Read the model definition and answer for the solid it produces. Units are mm, in the model's axes. A direction names the side the tool comes from. Round coordinates to 2 decimals unless told otherwise and drop trailing zeros. Loops run counter-clockwise (first coordinate to the right, second up) from the corner with the lowest first, then second, coordinate; pieces in that order, holes last. Notation, with made-up numbers: M 85.5,12.5 L 94.5,12.5 A18 cw 94.5,25.5 Z; hole C 38,68.5 d9. An arc over 180 degrees is marked long. Write each question's results on one line, items separated by ' | '.
from build123d import *

# Parameters (mm, degrees)
SKETCH1_R                = 14.5
BOSS_EXTRUDE1_DEPTH      = 4
BOSS_EXTRUDE2_DEPTH      = 2
BOSS_EXTRUDE2_DEPTH_BACK = 125
SKETCH2_R                = 5
SKETCH2_R_2              = 4
SKETCH2_R_3              = 3.453892414
SKETCH2_R_4              = 2.453892414
LPATTERN4_START          = -124
LPATTERN4_OUTLINE_R      = 14.5
LPATTERN4_DEPTH          = 4
LPATTERN4_START_2        = -62
LPATTERN4_2_OUTLINE_R    = 14.5
LPATTERN4_2_OUTLINE_R_2  = 3.453892414
LPATTERN4_2_OUTLINE_R_3  = 5
LPATTERN4_2_OUTLINE_R_4  = 4
LPATTERN4_2_OUTLINE_R_5  = 2.453892414
LPATTERN4_2_DEPTH        = 4
SKETCH8_R                = 2.453892414
CUT_EXTRUDE4_DEPTH       = 128
SKETCH12_R               = 2.875
BOSS_EXTRUDE4_DEPTH      = 41
CUT_EXTRUDE5_DEPTH       = 41
SKETCH14_R               = 4
CUT_EXTRUDE6_DEPTH       = 124


# Read off the part's stored shape, not the designer's step: LPattern4
with BuildPart() as part:
    # Sketch1 → Boss-Extrude1 (new body)
    with BuildSketch(Plane(origin=(0, 0, 0), x_dir=(1, 0, 0), z_dir=(0, 1, 0))):
        with Locations(Location((0, 0, 0), (0, 0, 270))):
            Circle(SKETCH1_R)
    extrude(amount=BOSS_EXTRUDE1_DEPTH)

    # Sketch2 → Boss-Extrude2 (add, two sides: drawn at the far end of the back side and taken through both)
    # profile 1 of 7: a face of its own
    with BuildSketch(Plane(origin=(0, 4, 0), x_dir=(1, 0, 0), z_dir=(0, 1, 0)).offset(-BOSS_EXTRUDE2_DEPTH_BACK)):
        with Locations(Location((0, 0, 0), (0, 0, 270))):
            Circle(SKETCH2_R)
        with Locations(Location((0, 0, 0), (0, 0, 270))):
            Circle(SKETCH2_R_2, mode=Mode.SUBTRACT)
    # profile 2 of 7: a face of its own
    with BuildSketch(Plane(origin=(0, 4, 0), x_dir=(1, 0, 0), z_dir=(0, 1, 0)).offset(-BOSS_EXTRUDE2_DEPTH_BACK)):
        with Locations(Location((0, 9.4, 0), (0, 0, 270))):
            Circle(SKETCH2_R_3)
        with Locations(Location((0, 9.4, 0), (0, 0, 270))):
            Circle(SKETCH2_R_4, mode=Mode.SUBTRACT)
    # profile 3 of 7: a face of its own
    with BuildSketch(Plane(origin=(0, 4, 0), x_dir=(1, 0, 0), z_dir=(0, 1, 0)).offset(-BOSS_EXTRUDE2_DEPTH_BACK)):
        with Locations(Location((8.140638796, 4.7, 0), (0, 0, 270))):
            Circle(SKETCH2_R_3)
        with Locations(Location((8.140638796, 4.7, 0), (0, 0, 270))):
            Circle(SKETCH2_R_4, mode=Mode.SUBTRACT)
    # profile 4 of 7: a face of its own
    with BuildSketch(Plane(origin=(0, 4, 0), x_dir=(1, 0, 0), z_dir=(0, 1, 0)).offset(-BOSS_EXTRUDE2_DEPTH_BACK)):
        with Locations(Location((8.140638796, -4.7, 0), (0, 0, 270))):
            Circle(SKETCH2_R_3)
        with Locations(Location((8.140638796, -4.7, 0), (0, 0, 270))):
            Circle(SKETCH2_R_4, mode=Mode.SUBTRACT)
    # profile 5 of 7: a face of its own
    with BuildSketch(Plane(origin=(0, 4, 0), x_dir=(1, 0, 0), z_dir=(0, 1, 0)).offset(-BOSS_EXTRUDE2_DEPTH_BACK)):
        with Locations(Location((0, -9.4, 0), (0, 0, 270))):
            Circle(SKETCH2_R_3)
        with Locations(Location((0, -9.4, 0), (0, 0, 270))):
            Circle(SKETCH2_R_4, mode=Mode.SUBTRACT)
    # profile 6 of 7: a face of its own
    with BuildSketch(Plane(origin=(0, 4, 0), x_dir=(1, 0, 0), z_dir=(0, 1, 0)).offset(-BOSS_EXTRUDE2_DEPTH_BACK)):
        with Locations(Location((-8.140638796, -4.7, 0), (0, 0, 270))):
            Circle(SKETCH2_R_3)
        with Locations(Location((-8.140638796, -4.7, 0), (0, 0, 270))):
            Circle(SKETCH2_R_4, mode=Mode.SUBTRACT)
    # profile 7 of 7: a face of its own
    with BuildSketch(Plane(origin=(0, 4, 0), x_dir=(1, 0, 0), z_dir=(0, 1, 0)).offset(-BOSS_EXTRUDE2_DEPTH_BACK)):
        with Locations(Location((-8.140638796, 4.7, 0), (0, 0, 270))):
            Circle(SKETCH2_R_3)
        with Locations(Location((-8.140638796, 4.7, 0), (0, 0, 270))):
            Circle(SKETCH2_R_4, mode=Mode.SUBTRACT)
    extrude(amount=BOSS_EXTRUDE2_DEPTH + BOSS_EXTRUDE2_DEPTH_BACK)

    # LPattern4 outline → LPattern4 (add)
    with BuildSketch(Plane(origin=(0, 0, 0), x_dir=(1, 0, 0), z_dir=(0, 1, 0)).offset(LPATTERN4_START)):
        Circle(LPATTERN4_OUTLINE_R)
    extrude(amount=LPATTERN4_DEPTH)

    # LPattern4 2 outline → LPattern4 2 (add)
    # profile 1 of 8: a face of its own
    with BuildSketch(Plane(origin=(0, 0, 0), x_dir=(1, 0, 0), z_dir=(0, 1, 0)).offset(LPATTERN4_START_2)):
        Circle(LPATTERN4_2_OUTLINE_R)
        with Locations((-8.140638796, -4.7)):
            Circle(LPATTERN4_2_OUTLINE_R_2, mode=Mode.SUBTRACT)
        with Locations((0, -9.4)):
            Circle(LPATTERN4_2_OUTLINE_R_2, mode=Mode.SUBTRACT)
        with Locations((8.140638796, -4.7)):
            Circle(LPATTERN4_2_OUTLINE_R_2, mode=Mode.SUBTRACT)
        with Locations((-8.140638796, 4.7)):
            Circle(LPATTERN4_2_OUTLINE_R_2, mode=Mode.SUBTRACT)
        Circle(LPATTERN4_2_OUTLINE_R_3, mode=Mode.SUBTRACT)
        with Locations((8.140638796, 4.7)):
            Circle(LPATTERN4_2_OUTLINE_R_2, mode=Mode.SUBTRACT)
        with Locations((0, 9.4)):
            Circle(LPATTERN4_2_OUTLINE_R_2, mode=Mode.SUBTRACT)
    # profile 2 of 8: a face of its own
    with BuildSketch(Plane(origin=(0, 0, 0), x_dir=(1, 0, 0), z_dir=(0, 1, 0)).offset(LPATTERN4_START_2)):
        Circle(LPATTERN4_2_OUTLINE_R_4)
    # profile 3 of 8: a face of its own
    with BuildSketch(Plane(origin=(0, 0, 0), x_dir=(1, 0, 0), z_dir=(0, 1, 0)).offset(LPATTERN4_START_2)):
        with Locations((0, 9.4)):
            Circle(LPATTERN4_2_OUTLINE_R_5)
    # profile 4 of 8: a face of its own
    with BuildSketch(Plane(origin=(0, 0, 0), x_dir=(1, 0, 0), z_dir=(0, 1, 0)).offset(LPATTERN4_START_2)):
        with Locations((8.140638796, 4.7)):
            Circle(LPATTERN4_2_OUTLINE_R_5)
    # profile 5 of 8: a face of its own
    with BuildSketch(Plane(origin=(0, 0, 0), x_dir=(1, 0, 0), z_dir=(0, 1, 0)).offset(LPATTERN4_START_2)):
        with Locations((8.140638796, -4.7)):
            Circle(LPATTERN4_2_OUTLINE_R_5)
    # profile 6 of 8: a face of its own
    with BuildSketch(Plane(origin=(0, 0, 0), x_dir=(1, 0, 0), z_dir=(0, 1, 0)).offset(LPATTERN4_START_2)):
        with Locations((0, -9.4)):
            Circle(LPATTERN4_2_OUTLINE_R_5)
    # profile 7 of 8: a face of its own
    with BuildSketch(Plane(origin=(0, 0, 0), x_dir=(1, 0, 0), z_dir=(0, 1, 0)).offset(LPATTERN4_START_2)):
        with Locations((-8.140638796, -4.7)):
            Circle(LPATTERN4_2_OUTLINE_R_5)
    # profile 8 of 8: a face of its own
    with BuildSketch(Plane(origin=(0, 0, 0), x_dir=(1, 0, 0), z_dir=(0, 1, 0)).offset(LPATTERN4_START_2)):
        with Locations((-8.140638796, 4.7)):
            Circle(LPATTERN4_2_OUTLINE_R_5)
    extrude(amount=LPATTERN4_2_DEPTH)

    # Sketch8 → Cut-Extrude4 (cut)
    with BuildSketch(Plane(origin=(0, 4, 0), x_dir=(1, 0, 0), z_dir=(0, 1, 0))):
        with Locations(Location((-8.140638796, -4.7, 0), (0, 0, 270))):
            Circle(SKETCH8_R)
        with Locations(Location((0, -9.4, 0), (0, 0, 270))):
            Circle(SKETCH8_R)
        with Locations(Location((8.140638796, -4.7, 0), (0, 0, 270))):
            Circle(SKETCH8_R)
        with Locations(Location((8.140638796, 4.7, 0), (0, 0, 270))):
            Circle(SKETCH8_R)
        with Locations(Location((0, 9.4, 0), (0, 0, 270))):
            Circle(SKETCH8_R)
        with Locations(Location((-8.140638796, 4.7, 0), (0, 0, 270))):
            Circle(SKETCH8_R)
    extrude(amount=-CUT_EXTRUDE4_DEPTH, mode=Mode.SUBTRACT)

    # Sketch12 → Boss-Extrude4 (add)
    with BuildSketch(Plane.XZ.offset(124)):
        with Locations(Location((0, 0, 0), (0, 0, 90))):
            Circle(SKETCH12_R)
    extrude(amount=BOSS_EXTRUDE4_DEPTH)

    # Sketch9 → Cut-Extrude5 (cut)
    with BuildSketch(Plane.XZ.offset(165)):
        with BuildLine():
            Line((1.5, 1.469693846), (1.5, -1.469693846))
            ThreePointArc((1.5, -1.469693846), (-2.1, 0), (1.5, 1.469693846))
        make_face()
    extrude(amount=-CUT_EXTRUDE5_DEPTH, mode=Mode.SUBTRACT)

    # Sketch14 → Cut-Extrude6 (cut)
    with BuildSketch(Plane(origin=(0, 4, 0), x_dir=(1, 0, 0), z_dir=(0, 1, 0))):
        with Locations(Location((0, 0, 0), (0, 0, 270))):
            Circle(SKETCH14_R)
    extrude(amount=-CUT_EXTRUDE6_DEPTH, mode=Mode.SUBTRACT)


solid = part.part
Item 1: Straight lines are drawn through the part: line 1 (Y direction, x = 2.5, z = -6.5); line 2 (X direction, y = 4.9, z = 0); line 3 (X direction, y = -82, z = 9.4). For each, find the intervals that lie inside material, in ascending order.
Outcome:
line 1: y = -124 to -120, -62 to -58, 0 to 4 | line 2: x = -5 to -4, 4 to 5 | line 3: x = -3.45 to -2.45, 2.45 to 3.45
Item 2: For faces 1 (the face through (1.037, 4.986, -6.106)), 2 (the face through (6, 6, -3)), 3 (the face through (1.037, -91.406, -6.106)), determine the directions among +Z, -Z, +X, -X, +Y, -Y from which every point of the face is accessible in a straight line to the end or side of a thin tool.
Outcome:
face 1: +Y | face 2: +Z, -Z, +X, -X, +Y | face 3: none
Item 3: The mould has two halves that part along Y. Classify faces 4 (the face through (1.5, -91.41, 4.77)), 5 (the face through (11.05, -91.41, 6.56)), 6 (the face through (-1, 6, -12)), 7 (the face through (-5.554, 1.972, 13.394)): pulls with the +Y half, pulls with the -Y half, needs draft (parallel to the pull), parting line crosses it, or undercut.
Outcome:
face 4: undercut | face 5: undercut | face 6: pulls with the +Y half | face 7: needs draft
Item 4: Flat-ended cylindrical pins translate along their axes: pin 1 (3 mm diameter, centred on x = 0, z = 9.4, fed in from -Y); pin 2 (8.5 mm diameter, centred on x = -6, z = 7, fed in from -Y); pin 3 (4 mm diameter, centred on x = 0.5, z = 0, fed in from +Y); pin 4 (4 mm diameter, centred on y = -114.5, z = 9, fed in from -X). Find the tip coordinate at first contact, or state that the pin passes through.
Outcome:
pin 1: passes through | pin 2: stops at y = -124 | pin 3: stops at y = -120 | pin 4: stops at x = -10.72
Item 5: The part is cut by section C-C (y = -132.5). Determine the outline of the cut face in (x, z) (3 decimals).
Outcome:
outline: C 0,0 d5.75; hole M 1.5,-1.47 L 1.5,1.47 A2.1 ccw long Z
Item 6: The part is cut by section A-A (y = -113.5). State how many separate pieces and enclosed holes the cut face has, plus the area to 3 significant figures.
Outcome:
separate pieces: 7 | enclosed holes: 7 | area: 140 mm2
